Verification items for the finished model (mm, model axes). A direction names the side the tool comes from. Coordinates: 2 decimals unless noted, no trailing zeros. Answer as CSV lines item,"result". Start each with the question number.
```python
from build123d import *

# Parameters (mm, degrees)
BOSS_EXTRUDE1_DEPTH      = 2
BOSS_EXTRUDE1_DEPTH_BACK = 7
BOSS_EXTRUDE3_DEPTH      = 9
SKETCH6_R                = 7
SKETCH6_R_2              = 3.69685312
BOSS_EXTRUDE4_DEPTH      = 3
BOSS_EXTRUDE5_DEPTH      = 38
SKETCH8_R                = 7
BOSS_EXTRUDE6_DEPTH      = 10
SKETCH9_R                = 7
SKETCH9_R_2              = 3.591571222
BOSS_EXTRUDE7_DEPTH      = 3
SKETCH10_R               = 7
CUT_EXTRUDE1_DEPTH       = 5.5
SKETCH11_R               = 3.591571222
CUT_EXTRUDE2_DEPTH       = 71.546467667


with BuildPart() as part:
    # Sketch2 → Boss-Extrude1 (new, two sides: drawn at the far end of the back side and taken through both)
    with BuildSketch(Plane.XY.offset(-BOSS_EXTRUDE1_DEPTH_BACK)):
        with BuildLine():
            Line((17.593003447, 3.447921134), (18.432689254, 3.812129579))
            ThreePointArc((18.432689254, 3.812129579), (18.142308848, 4.822341152), (17.760116965, 5.801513031))
            Line((17.760116965, 5.801513031), (16.871688472, 5.581479263))
            Line((16.871688472, 5.581479263), (15.649099733, 5.241598415))
            ThreePointArc((15.649099733, 5.241598415), (15.22663553, 6.009376293), (14.733410626, 6.733729845))
            Line((14.733410626, 6.733729845), (15.590096731, 7.669855443))
            Line((15.590096731, 7.669855443), (16.188603379, 8.362321932))
            ThreePointArc((16.188603379, 8.362321932), (15.488665299, 9.146499772), (14.719475556, 9.862876308))
            Line((14.719475556, 9.862876308), (14.014498216, 9.279158058))
            Line((14.014498216, 9.279158058), (13.060452596, 8.442474621))
            ThreePointArc((13.060452596, 8.442474621), (12.346699165, 8.950918239), (11.588033655, 9.389535972))
            Line((11.588033655, 9.389535972), (11.95371149, 10.604658163))
            Line((11.95371149, 10.604658163), (12.192497398, 11.488231214))
            ThreePointArc((12.192497398, 11.488231214), (11.221632964, 11.891059284), (10.217792822, 12.202753318))
            Line((10.217792822, 12.202753318), (9.835896044, 11.370963143))
            Line((9.835896044, 11.370963143), (9.33935398, 10.203192533))
            ThreePointArc((9.33935398, 10.203192533), (8.475678941, 10.351598396), (7.601835833, 10.417606691))
            Line((7.601835833, 10.417606691), (7.404078418, 11.671055622))
            Line((7.404078418, 11.671055622), (7.235849109, 12.570732756))
            ThreePointArc((7.235849109, 12.570732756), (6.18634993, 12.512426015), (5.14668224, 12.357702722))
            Line((5.14668224, 12.357702722), (5.163505363, 11.442586867))
            Line((5.163505363, 11.442586867), (5.222813101, 10.175020376))
            ThreePointArc((5.222813101, 10.175020376), (4.380277888, 9.933994883), (3.564332526, 9.614319987))
            Line((3.564332526, 9.614319987), (2.842308143, 10.657834724))
            Line((2.842308143, 10.657834724), (2.300383494, 11.395423851))
            ThreePointArc((2.300383494, 11.395423851), (1.380115753, 10.887530665), (0.510539453, 10.297034891))
            Line((0.510539453, 10.297034891), (0.922750452, 9.479843274))
            Line((0.922750452, 9.479843274), (1.526161366, 8.363537991))
            ThreePointArc((1.526161366, 8.363537991), (0.871640411, 7.780819197), (0.275200782, 7.138776643))
            Line((0.275200782, 7.138776643), (-0.828084785, 7.765676295))
            Line((-0.828084785, 7.765676295), (-1.636369952, 8.195088843))
            ThreePointArc((-1.636369952, 8.195088843), (-2.245135941, 7.338203686), (-2.772390602, 6.42889036))
            Line((-2.772390602, 6.42889036), (-2.04643517, 5.871477804))
            Line((-2.04643517, 5.871477804), (-1.018434012, 5.12753168))
            ThreePointArc((-1.018434012, 5.12753168), (-1.355304806, 4.318534189), (-1.61410652, 3.481288379))
            Line((-1.61410652, 3.481288379), (-2.880134034, 3.567407782))
            Line((-2.880134034, 3.567407782), (-3.794688927, 3.603593329))
            ThreePointArc((-3.794688927, 3.603593329), (-3.971379595, 2.567432815), (-4.051883364, 1.519402593))
            Line((-4.051883364, 1.519402593), (-3.155967876, 1.332171491))
            Line((-3.155967876, 1.332171491), (-1.90698471, 1.107932181))
            ThreePointArc((-1.90698471, 1.107932181), (-1.859483953, 0.232887867), (-1.729388897, -0.633734398))
            Line((-1.729388897, -0.633734398), (-2.907406081, -1.105452248))
            Line((-2.907406081, -1.105452248), (-3.747091888, -1.469660694))
            ThreePointArc((-3.747091888, -1.469660694), (-3.456711482, -2.479872267), (-3.0745196, -3.459044145))
            Line((-3.0745196, -3.459044145), (-2.186091107, -3.239010378))
            Line((-2.186091107, -3.239010378), (-0.963502367, -2.899129529))
            ThreePointArc((-0.963502367, -2.899129529), (-0.541038164, -3.666907408), (-0.047813261, -4.391260959))
            Line((-0.047813261, -4.391260959), (-0.904499365, -5.327386558))
            Line((-0.904499365, -5.327386558), (-1.503006014, -6.019853046))
            ThreePointArc((-1.503006014, -6.019853046), (-0.803067933, -6.804030887), (-0.03387819, -7.520407423))
            Line((-0.03387819, -7.520407423), (0.67109915, -6.936689172))
            Line((0.67109915, -6.936689172), (1.625144769, -6.100005735))
            ThreePointArc((1.625144769, -6.100005735), (2.3388982, -6.608449353), (3.097563711, -7.047067087))
            Line((3.097563711, -7.047067087), (2.731885876, -8.262189278))
            Line((2.731885876, -8.262189278), (2.493099968, -9.145762328))
            ThreePointArc((2.493099968, -9.145762328), (3.463964401, -9.548590398), (4.467804544, -9.860284433))
            Line((4.467804544, -9.860284433), (4.849701322, -9.028494257))
            Line((4.849701322, -9.028494257), (5.346243386, -7.860723648))
            ThreePointArc((5.346243386, -7.860723648), (6.209918425, -8.009129511), (7.083761533, -8.075137806))
            Line((7.083761533, -8.075137806), (7.281518948, -9.328586736))
            Line((7.281518948, -9.328586736), (7.449748257, -10.22826387))
            ThreePointArc((7.449748257, -10.22826387), (8.499247436, -10.16995713), (9.538915126, -10.015233837))
            Line((9.538915126, -10.015233837), (9.522092003, -9.100117982))
            Line((9.522092003, -9.100117982), (9.462784265, -7.83255149))
            ThreePointArc((9.462784265, -7.83255149), (10.305319478, -7.591525998), (11.12126484, -7.271851101))
            Line((11.12126484, -7.271851101), (11.843289223, -8.315365839))
            Line((11.843289223, -8.315365839), (12.385213872, -9.052954966))
            ThreePointArc((12.385213872, -9.052954966), (13.305481612, -8.54506178), (14.175057913, -7.954566005))
            Line((14.175057913, -7.954566005), (13.762846914, -7.137374389))
            Line((13.762846914, -7.137374389), (13.159436, -6.021069105))
            ThreePointArc((13.159436, -6.021069105), (13.813956955, -5.438350311), (14.410396584, -4.796307757))
            Line((14.410396584, -4.796307757), (15.513682151, -5.42320741))
            Line((15.513682151, -5.42320741), (16.321967317, -5.852619957))
            ThreePointArc((16.321967317, -5.852619957), (16.930733307, -4.9957348), (17.457987967, -4.086421474))
            Line((17.457987967, -4.086421474), (16.732032536, -3.529008918))
            Line((16.732032536, -3.529008918), (15.704031377, -2.785062794))
            ThreePointArc((15.704031377, -2.785062794), (16.040902172, -1.976065303), (16.299703886, -1.138819493))
            Line((16.299703886, -1.138819493), (17.565731399, -1.224938896))
            Line((17.565731399, -1.224938896), (18.480286292, -1.261124443))
            ThreePointArc((18.480286292, -1.261124443), (18.656976961, -0.22496393), (18.737480729, 0.823066292))
            Line((18.737480729, 0.823066292), (17.841565242, 1.010297394))
            Line((17.841565242, 1.010297394), (16.592582076, 1.234536705))
            ThreePointArc((16.592582076, 1.234536705), (16.545081318, 2.109581019), (16.414986263, 2.976203284))
            Line((16.414986263, 2.976203284), (17.593003447, 3.447921134))
        make_face()
    extrude(amount=BOSS_EXTRUDE1_DEPTH + BOSS_EXTRUDE1_DEPTH_BACK)

    # Sketch5 → Boss-Extrude3 (add)
    with BuildSketch(Plane.XY.offset(2)):
        with BuildLine():
            Line((14.323069399, -7.330284288), (11.497184032, -4.736041982))
            Line((11.497184032, -4.736041982), (2.348634103, -4.736041982))
            add(Edge.make_bspline(
                [(2.348634103, -4.736041982), (0.628552499, -19.32789347), (-1.912663, -35.361500183), (4.763482553, -49.160053836)],
                knots=[0, 0, 0, 0, 1, 1, 1, 1], degree=3))
            Line((4.763482553, -49.160053836), (10.332905106, -48.613760737))
            Line((10.332905106, -48.613760737), (7.574511186, -24.888738823))
            add(Edge.make_bspline(
                [(14.323069399, -7.330284288), (7.759285057, -14.975557189), (7.574511186, -24.888738823)],
                knots=[0, 0, 0, 1, 1, 1], degree=2))
        make_face()
    extrude(amount=-BOSS_EXTRUDE3_DEPTH)

    # Sketch6 → Boss-Extrude4 (add)
    with BuildSketch(Plane(origin=(0, 0, -7), x_dir=(-1, 0, 0), z_dir=(0, 0, -1))):
        with Locations((-7.342798683, 1.171234443)):
            Circle(SKETCH6_R)
        with Locations((-7.342798683, 1.171234443)):
            Circle(SKETCH6_R_2, mode=Mode.SUBTRACT)
    extrude(amount=-BOSS_EXTRUDE4_DEPTH)

    # Sketch7 → Boss-Extrude5 (add)
    with BuildSketch(Plane.XY.offset(2)):
        with BuildLine():
            Line((4.763482553, -49.160053836), (10.332905106, -48.613760737))
            Line((10.332905106, -48.613760737), (7.574511187, -24.888738781))
            add(Edge.make_bspline(
                [(7.574511187, -24.888738781), (7.686436039, -21.137993885), (8.653774634, -17.660128373)],
                knots=[0, 0, 0, 1, 1, 1], degree=2))
            add(Edge.make_bspline(
                [(0.854001662, -18.172152661), (4.511582235, -11.66623094), (8.653774634, -17.660128373)],
                knots=[0, 0, 0, 1, 1, 1], degree=2))
            add(Edge.make_bspline(
                [(0.854001662, -18.172152661), (-0.132777517, -28.73684408), (0.123220881, -39.513312679), (4.763482553, -49.160053836)],
                knots=[0.2758018, 0.2758018, 0.2758018, 0.2758018, 1, 1, 1, 1], degree=3))
        make_face()
    extrude(amount=BOSS_EXTRUDE5_DEPTH)

    # Sketch8 → Boss-Extrude6 (add)
    with BuildSketch(Plane.XY.offset(40)):
        with BuildLine():
            add(Edge.make_bspline(
                [(8.161452368, -19.485656093), (9.314674226, -14.585302427), (12.103080861, -10.251209775)],
                knots=[0, 0, 0, 1, 1, 1], degree=2))
            add(Edge.make_bspline(
                [(1.784517867, -9.294701523), (-1.285057106, -6.227479148), (-7.467073574, 5.277430619), (17.020799468, 17.744922671), (19.383717346, -6.805513304), (12.103080861, -10.251209775)],
                knots=[0, 0, 0, 0, 0.273426671, 0.5551446, 1, 1, 1, 1], degree=3))
            add(Edge.make_bspline(
                [(1.784517867, -9.294701523), (1.392693521, -12.484419655), (1.032610994, -15.724984195), (0.780859851, -18.982230478)],
                knots=[0.071303054, 0.071303054, 0.071303054, 0.071303054, 0.275801801, 0.275801801, 0.275801801, 0.275801801], degree=3))
            add(Edge.make_bspline(
                [(0.780859851, -18.982230478), (4.753063038, -11.185515123), (8.161452368, -19.485656093)],
                knots=[0, 0, 0, 1, 1, 1], degree=2))
        make_face()
        with Locations((7.342798683, 1.171234443)):
            Circle(SKETCH8_R, mode=Mode.SUBTRACT)
    extrude(amount=-BOSS_EXTRUDE6_DEPTH)

    # Sketch9 → Boss-Extrude7 (add)
    with BuildSketch(Plane.XY.offset(40)):
        with Locations((7.342798683, 1.171234443)):
            Circle(SKETCH9_R)
        with Locations((7.342798683, 1.171234443)):
            Circle(SKETCH9_R_2, mode=Mode.SUBTRACT)
    extrude(amount=-BOSS_EXTRUDE7_DEPTH)

    # Sketch10 → Cut-Extrude1 (cut)
    with BuildSketch(Plane.XY.offset(2)):
        with Locations((7.342798683, 1.171234443)):
            Circle(SKETCH10_R)
    extrude(amount=-CUT_EXTRUDE1_DEPTH, mode=Mode.SUBTRACT)

    # Sketch11 → Cut-Extrude2 (cut, through all)
    with BuildSketch(Plane(origin=(0, 0, -7), x_dir=(-1, 0, 0), z_dir=(0, 0, -1))):
        with Locations(Location((-7.342798683, 1.171234443, 0), (0, 0, 180))):
            Circle(SKETCH11_R)
    extrude(amount=-CUT_EXTRUDE2_DEPTH, mode=Mode.SUBTRACT)


solid = part.part
```
1. Access from +Z, -Z, +X, -X, +Y, -Y to the whole of each face (thin tool, end or side, straight path). Record for faces 3 (the face through (-2.54, 1.22, -2.56)), 4 (the face through (-2.238, 3.524, -2.563)), 5 (the face through (16.546, 2.097, -2.563)).
2. Draft check along Z on faces 1 (the face through (12.36, 8.94, -2.56)), 2 (the face through (4, 3, -3.5)). Enter one of: pulls with the +Z half, pulls with the -Z half, needs draft (parallel to the pull), parting line crosses it, or undercut.
3. Depth check by flat-ended pin: P1, Ø0.5, axis at x = 8, y = -21, coming from the -Z side; P2, Ø8, axis at y = -7.5, z = 32.5, coming from the +X side; P3, Ø1.5, axis at x = 6, z = 9.5, coming from the -Y side; P4, Ø10, axis at y = -12.5, z = 27, coming from the -X side. Enter the tip coordinate at first touch or a pass-through.
4. Scan lines: line 1 along Z through (x, y) = (12, -8.5); line 2 along Y through (x, z) = (15, -1.5); line 3 along Y through (x, z) = (15.5, -1). Record each from-to range of solid material in increasing order. Write a range as from..to.
Completed:
1,face 3,"-Z, -X"
1,face 4,"-Z"
1,face 5,"-Z, +X"
2,face 1,"needs draft"
2,face 2,"undercut"
3,P1,"stops at z = -7"
3,P2,"stops at x = 16.65"
3,P3,"stops at y = -49.11"
3,P4,"stops at x = 0.99"
4,line 1,"z = -7..2, 30..40"
4,line 2,"y = -5.13..6.36, 7.03..9.62"
4,line 3,"y = -5.42..5.53, 7.57..9.13"
